from build123d import *
from OCP.BRepFilletAPI import BRepFilletAPI_MakeChamfer

# Parameters (mm, degrees)
BASE_SKETCH_W          = 50
BASE_SKETCH_H          = 50
BASE_EXTRUDE_DEPTH     = 5
CIRCLES_SKETCH_R       = 1.5
CIRCLE_CUTS_DEPTH      = 5
EDGE_FILLET_R          = 0.5
CIRCULAR_CHAMFER_SIZE  = 0.25
CIRCULAR_CHAMFER_SIZE2 = 0.144337567


with BuildPart() as part:
    # Base Sketch → Base Extrude (new body)
    with BuildSketch(Plane(origin=(0, 0, 0), x_dir=(1, 0, 0), z_dir=(0, 1, 0))):
        Rectangle(BASE_SKETCH_W, BASE_SKETCH_H)
    extrude(amount=BASE_EXTRUDE_DEPTH)

    # Circles Sketch → Circle Cuts (cut)
    with BuildSketch(Plane(origin=(0, 5, 0), x_dir=(1, 0, 0), z_dir=(0, 1, 0))):
        with Locations(Location((-18.75, 18.75, 0), (0, 0, 270))):
            Circle(CIRCLES_SKETCH_R)
        with Locations(Location((-6.25, 18.75, 0), (0, 0, 270))):
            Circle(CIRCLES_SKETCH_R)
        with Locations(Location((6.25, 18.75, 0), (0, 0, 270))):
            Circle(CIRCLES_SKETCH_R)
        with Locations(Location((18.75, 18.75, 0), (0, 0, 270))):
            Circle(CIRCLES_SKETCH_R)
        with Locations(Location((-18.75, 6.25, 0), (0, 0, 270))):
            Circle(CIRCLES_SKETCH_R)
        with Locations(Location((-6.25, 6.25, 0), (0, 0, 270))):
            Circle(CIRCLES_SKETCH_R)
        with Locations(Location((6.25, 6.25, 0), (0, 0, 270))):
            Circle(CIRCLES_SKETCH_R)
        with Locations(Location((18.75, 6.25, 0), (0, 0, 270))):
            Circle(CIRCLES_SKETCH_R)
        with Locations(Location((-18.75, -6.25, 0), (0, 0, 270))):
            Circle(CIRCLES_SKETCH_R)
        with Locations(Location((-6.25, -6.25, 0), (0, 0, 270))):
            Circle(CIRCLES_SKETCH_R)
        with Locations(Location((6.25, -6.25, 0), (0, 0, 270))):
            Circle(CIRCLES_SKETCH_R)
        with Locations(Location((18.75, -6.25, 0), (0, 0, 270))):
            Circle(CIRCLES_SKETCH_R)
        with Locations(Location((-18.75, -18.75, 0), (0, 0, 270))):
            Circle(CIRCLES_SKETCH_R)
        with Locations(Location((-6.25, -18.75, 0), (0, 0, 270))):
            Circle(CIRCLES_SKETCH_R)
        with Locations(Location((6.25, -18.75, 0), (0, 0, 270))):
            Circle(CIRCLES_SKETCH_R)
        with Locations(Location((18.75, -18.75, 0), (0, 0, 270))):
            Circle(CIRCLES_SKETCH_R)
    extrude(amount=-CIRCLE_CUTS_DEPTH, mode=Mode.SUBTRACT)

    # Edge Fillet
    edge_fillet_edges = [part.edges().sort_by_distance(p)[0] for p in [
        (-25, 5, 0),
        (0, 5, 25),
        (25, 5, 0),
        (0, 0, 25),
        (-25, 0, 0),
        (0, 0, -25),
        (25, 0, 0),
        (25, 2.5, 25),
        (-25, 2.5, 25),
        (-25, 2.5, -25),
        (25, 2.5, -25),
        (0, 5, -25),
    ]]
    fillet(edge_fillet_edges, radius=EDGE_FILLET_R)

    # Circular Chamfer: one chamfer whose edges measure the first distance from different faces: ONE call of the kernel's chamfer builder (chamfer() names one face for all edges)
    circular_chamfer_edges_1 = [part.edges().sort_by_distance(p)[0] for p in [
        (18.75, 0, -20.25),
    ]]
    circular_chamfer_side_1 = [part.faces().sort_by_distance(p)[0] for p in [
        (18.75, 2.5, -20.25),
    ]]
    circular_chamfer_edges_2 = [part.edges().sort_by_distance(p)[0] for p in [
        (18.75, 5, -20.25),
        (6.25, 5, -20.25),
        (6.25, 5, -7.75),
        (6.25, 5, 4.75),
        (-6.25, 5, 4.75),
        (-6.25, 5, -7.75),
        (-6.25, 5, -20.25),
        (-18.75, 5, -20.25),
        (-18.75, 5, 17.25),
        (-6.25, 5, 17.25),
        (6.25, 5, 17.25),
        (18.75, 5, 4.75),
        (18.75, 5, 17.25),
        (-18.75, 5, 4.75),
        (-18.75, 5, -7.75),
        (18.75, 5, -7.75),
    ]]
    circular_chamfer_side_2 = [part.faces().sort_by_distance(p)[0] for p in [
        (0, 5, 0),
    ]]
    circular_chamfer_edges_3 = [part.edges().sort_by_distance(p)[0] for p in [
        (6.25, 0, -20.25),
    ]]
    circular_chamfer_side_3 = [part.faces().sort_by_distance(p)[0] for p in [
        (6.25, 2.5, -20.25),
    ]]
    circular_chamfer_edges_4 = [part.edges().sort_by_distance(p)[0] for p in [
        (6.25, 0, -7.75),
    ]]
    circular_chamfer_side_4 = [part.faces().sort_by_distance(p)[0] for p in [
        (6.25, 2.5, -7.75),
    ]]
    circular_chamfer_edges_5 = [part.edges().sort_by_distance(p)[0] for p in [
        (6.25, 0, 4.75),
    ]]
    circular_chamfer_side_5 = [part.faces().sort_by_distance(p)[0] for p in [
        (6.25, 2.5, 4.75),
    ]]
    circular_chamfer_edges_6 = [part.edges().sort_by_distance(p)[0] for p in [
        (-6.25, 0, 4.75),
    ]]
    circular_chamfer_side_6 = [part.faces().sort_by_distance(p)[0] for p in [
        (-6.25, 2.5, 4.75),
    ]]
    circular_chamfer_edges_7 = [part.edges().sort_by_distance(p)[0] for p in [
        (-6.25, 0, -7.75),
    ]]
    circular_chamfer_side_7 = [part.faces().sort_by_distance(p)[0] for p in [
        (-6.25, 2.5, -7.75),
    ]]
    circular_chamfer_edges_8 = [part.edges().sort_by_distance(p)[0] for p in [
        (-6.25, 0, -20.25),
    ]]
    circular_chamfer_side_8 = [part.faces().sort_by_distance(p)[0] for p in [
        (-6.25, 2.5, -20.25),
    ]]
    circular_chamfer_edges_9 = [part.edges().sort_by_distance(p)[0] for p in [
        (-18.75, 0, -20.25),
    ]]
    circular_chamfer_side_9 = [part.faces().sort_by_distance(p)[0] for p in [
        (-18.75, 2.5, -20.25),
    ]]
    circular_chamfer_edges_10 = [part.edges().sort_by_distance(p)[0] for p in [
        (-18.75, 0, 17.25),
    ]]
    circular_chamfer_side_10 = [part.faces().sort_by_distance(p)[0] for p in [
        (-18.75, 2.5, 17.25),
    ]]
    circular_chamfer_edges_11 = [part.edges().sort_by_distance(p)[0] for p in [
        (-6.25, 0, 17.25),
    ]]
    circular_chamfer_side_11 = [part.faces().sort_by_distance(p)[0] for p in [
        (-6.25, 2.5, 17.25),
    ]]
    circular_chamfer_edges_12 = [part.edges().sort_by_distance(p)[0] for p in [
        (6.25, 0, 17.25),
    ]]
    circular_chamfer_side_12 = [part.faces().sort_by_distance(p)[0] for p in [
        (6.25, 2.5, 17.25),
    ]]
    circular_chamfer_edges_13 = [part.edges().sort_by_distance(p)[0] for p in [
        (18.75, 0, 4.75),
    ]]
    circular_chamfer_side_13 = [part.faces().sort_by_distance(p)[0] for p in [
        (18.75, 2.5, 4.75),
    ]]
    circular_chamfer_edges_14 = [part.edges().sort_by_distance(p)[0] for p in [
        (18.75, 0, 17.25),
    ]]
    circular_chamfer_side_14 = [part.faces().sort_by_distance(p)[0] for p in [
        (18.75, 2.5, 17.25),
    ]]
    circular_chamfer_edges_15 = [part.edges().sort_by_distance(p)[0] for p in [
        (-18.75, 0, 4.75),
    ]]
    circular_chamfer_side_15 = [part.faces().sort_by_distance(p)[0] for p in [
        (-18.75, 2.5, 4.75),
    ]]
    circular_chamfer_edges_16 = [part.edges().sort_by_distance(p)[0] for p in [
        (-18.75, 0, -7.75),
    ]]
    circular_chamfer_side_16 = [part.faces().sort_by_distance(p)[0] for p in [
        (-18.75, 2.5, -7.75),
    ]]
    circular_chamfer_edges_17 = [part.edges().sort_by_distance(p)[0] for p in [
        (18.75, 0, -7.75),
    ]]
    circular_chamfer_side_17 = [part.faces().sort_by_distance(p)[0] for p in [
        (18.75, 2.5, -7.75),
    ]]
    circular_chamfer = BRepFilletAPI_MakeChamfer(part.part.solid().wrapped)
    for e in circular_chamfer_edges_1:
        circular_chamfer.Add(CIRCULAR_CHAMFER_SIZE, CIRCULAR_CHAMFER_SIZE2, e.wrapped, circular_chamfer_side_1[0].wrapped)  # the first distance lies on this face
    for e in circular_chamfer_edges_2:
        circular_chamfer.Add(CIRCULAR_CHAMFER_SIZE, CIRCULAR_CHAMFER_SIZE2, e.wrapped, circular_chamfer_side_2[0].wrapped)  # the first distance lies on this face
    for e in circular_chamfer_edges_3:
        circular_chamfer.Add(CIRCULAR_CHAMFER_SIZE, CIRCULAR_CHAMFER_SIZE2, e.wrapped, circular_chamfer_side_3[0].wrapped)  # the first distance lies on this face
    for e in circular_chamfer_edges_4:
        circular_chamfer.Add(CIRCULAR_CHAMFER_SIZE, CIRCULAR_CHAMFER_SIZE2, e.wrapped, circular_chamfer_side_4[0].wrapped)  # the first distance lies on this face
    for e in circular_chamfer_edges_5:
        circular_chamfer.Add(CIRCULAR_CHAMFER_SIZE, CIRCULAR_CHAMFER_SIZE2, e.wrapped, circular_chamfer_side_5[0].wrapped)  # the first distance lies on this face
    for e in circular_chamfer_edges_6:
        circular_chamfer.Add(CIRCULAR_CHAMFER_SIZE, CIRCULAR_CHAMFER_SIZE2, e.wrapped, circular_chamfer_side_6[0].wrapped)  # the first distance lies on this face
    for e in circular_chamfer_edges_7:
        circular_chamfer.Add(CIRCULAR_CHAMFER_SIZE, CIRCULAR_CHAMFER_SIZE2, e.wrapped, circular_chamfer_side_7[0].wrapped)  # the first distance lies on this face
    for e in circular_chamfer_edges_8:
        circular_chamfer.Add(CIRCULAR_CHAMFER_SIZE, CIRCULAR_CHAMFER_SIZE2, e.wrapped, circular_chamfer_side_8[0].wrapped)  # the first distance lies on this face
    for e in circular_chamfer_edges_9:
        circular_chamfer.Add(CIRCULAR_CHAMFER_SIZE, CIRCULAR_CHAMFER_SIZE2, e.wrapped, circular_chamfer_side_9[0].wrapped)  # the first distance lies on this face
    for e in circular_chamfer_edges_10:
        circular_chamfer.Add(CIRCULAR_CHAMFER_SIZE, CIRCULAR_CHAMFER_SIZE2, e.wrapped, circular_chamfer_side_10[0].wrapped)  # the first distance lies on this face
    for e in circular_chamfer_edges_11:
        circular_chamfer.Add(CIRCULAR_CHAMFER_SIZE, CIRCULAR_CHAMFER_SIZE2, e.wrapped, circular_chamfer_side_11[0].wrapped)  # the first distance lies on this face
    for e in circular_chamfer_edges_12:
        circular_chamfer.Add(CIRCULAR_CHAMFER_SIZE, CIRCULAR_CHAMFER_SIZE2, e.wrapped, circular_chamfer_side_12[0].wrapped)  # the first distance lies on this face
    for e in circular_chamfer_edges_13:
        circular_chamfer.Add(CIRCULAR_CHAMFER_SIZE, CIRCULAR_CHAMFER_SIZE2, e.wrapped, circular_chamfer_side_13[0].wrapped)  # the first distance lies on this face
    for e in circular_chamfer_edges_14:
        circular_chamfer.Add(CIRCULAR_CHAMFER_SIZE, CIRCULAR_CHAMFER_SIZE2, e.wrapped, circular_chamfer_side_14[0].wrapped)  # the first distance lies on this face
    for e in circular_chamfer_edges_15:
        circular_chamfer.Add(CIRCULAR_CHAMFER_SIZE, CIRCULAR_CHAMFER_SIZE2, e.wrapped, circular_chamfer_side_15[0].wrapped)  # the first distance lies on this face
    for e in circular_chamfer_edges_16:
        circular_chamfer.Add(CIRCULAR_CHAMFER_SIZE, CIRCULAR_CHAMFER_SIZE2, e.wrapped, circular_chamfer_side_16[0].wrapped)  # the first distance lies on this face
    for e in circular_chamfer_edges_17:
        circular_chamfer.Add(CIRCULAR_CHAMFER_SIZE, CIRCULAR_CHAMFER_SIZE2, e.wrapped, circular_chamfer_side_17[0].wrapped)  # the first distance lies on this face
    add(Compound.cast(circular_chamfer.Shape()), mode=Mode.REPLACE)


solid = part.part
For this review, take the finished solid that the model builds, in its own axes (mm). Give positions to 0.01 mm unless a question says otherwise; leave off trailing zeros. Answer in a Markdown table with one row per item. Add a question column.
(1) For pin 1 (2.5 mm diameter, centred on x = -18.75, z = 6.25, fed in from +Y), flat-tipped, find the tip position at first contact; note if it passes through.
(2) Consider section A-A on y = 2.5. Give the number of separate pieces and of enclosed holes in the cut face, and give its area (3 significant figures).
(3) Mouldability with a two-part tool opening along Z and no side actions: class faces 1 (the face through (6.32, 2.59, -7.75)), 2 (the face through (0, 0, 0)), 3 (the face through (19.76, 2.59, 17.64)) as +Z half, -Z half, draft (parallel to the pull), parting line (faces both ways), or undercut.
(4) Wall thickness on probe 1 along X at (y, z) = (3.5, -18.75); probe 2 along Z at (x, y) = (6.5, 3.1); probe 3 along X at (y, z) = (1.05, -7): over which ranges is each line inside the solid? List them lowest first. Write a range as [from, to].
Evaluation:
| question | item | result |
|---|---|---|
| 1 | pin 1 | passes through |
| 2 | separate pieces | 1 |
| 2 | enclosed holes | 16 |
| 2 | area | 2,390 mm^2 |
| 3 | face 1 | undercut |
| 3 | face 2 | draft |
| 3 | face 3 | undercut |
| 4 | probe 1 | x = [-25, -20.25], [-17.25, -7.75], [-4.75, 4.75], [7.75, 17.25], [20.25, 25] |
| 4 | probe 2 | z = [-25, -20.23], [-17.27, -7.73], [-4.77, 4.77], [7.73, 17.27], [20.23, 25] |
| 4 | probe 3 | x = [-25, -20.05], [-17.45, -7.55], [-4.95, 4.95], [7.55, 17.45], [20.05, 25] |
